```python
from build123d import *

# Parameters (mm, degrees)
SKETCH1_R               = 8.382
BOSS_EXTRUDE1_DEPTH     = 7.62
SKETCH2_R               = 5.588
BOSS_EXTRUDE2_DEPTH     = 7.112
SKETCH3_R               = 8.382
BOSS_EXTRUDE3_DEPTH     = 1.27
SKETCH4_R               = 2.54
CUT_EXTRUDE1_DEPTH      = 1
CUT_EXTRUDE1_DEPTH_BACK = 17.002
CHAMFER1_SIZE           = 0.508
SKETCH5_R               = 1.651
CUT_EXTRUDE2_DEPTH      = 9.382


with BuildPart() as part:
    # Sketch1 → Boss-Extrude1 (new body)
    with BuildSketch(Plane(origin=(0, 0, 0), x_dir=(1, 0, 0), z_dir=(0, 1, 0))):
        Circle(SKETCH1_R)
    extrude(amount=-BOSS_EXTRUDE1_DEPTH)

    # Sketch2 → Boss-Extrude2 (add)
    with BuildSketch(Plane(origin=(0, 0, 0), x_dir=(1, 0, 0), z_dir=(0, 1, 0))):
        with BuildLine():
            ThreePointArc((-4.121307864, 3.77366738), (-4.666752119, 3.721610627), (-4.596130935, 3.178258081))
            ThreePointArc((-4.596130935, 3.178258081), (-4.368874324, 3.484061013), (-4.121307864, 3.77366738))
        make_face()
        with BuildLine():
            ThreePointArc((-4.857698061, 2.761976385), (-5.377883173, 2.589852039), (-5.188125293, 2.075837167))
            ThreePointArc((-5.188125293, 2.075837167), (-5.034614034, 2.424542334), (-4.857698061, 2.761976385))
        make_face()
        with BuildLine():
            ThreePointArc((-5.350502993, 1.611788361), (-5.819344708, 1.328227455), (-5.519965385, 0.86932511))
            ThreePointArc((-5.519965385, 0.86932511), (-5.447897173, 1.243446979), (-5.350502993, 1.611788361))
        make_face()
        with BuildLine():
            ThreePointArc((-5.575011364, 0.380778538), (-5.969, 0), (-5.575011364, -0.380778538))
            ThreePointArc((-5.575011364, -0.380778538), (-5.588, 0), (-5.575011364, 0.380778538))
        make_face()
        with BuildLine():
            ThreePointArc((-5.350502993, -1.611788361), (-5.447897173, -1.243446979), (-5.519965385, -0.86932511))
            ThreePointArc((-5.519965385, -0.86932511), (-5.819344708, -1.328227455), (-5.350502993, -1.611788361))
        make_face()
        with BuildLine():
            ThreePointArc((-4.857698061, -2.761976385), (-5.034614034, -2.424542334), (-5.188125293, -2.075837167))
            ThreePointArc((-5.188125293, -2.075837167), (-5.377883173, -2.589852039), (-4.857698061, -2.761976385))
        make_face()
        with BuildLine():
            ThreePointArc((-4.121307864, -3.77366738), (-4.368874324, -3.484061013), (-4.596130935, -3.178258081))
            ThreePointArc((-4.596130935, -3.178258081), (-4.666752119, -3.721610627), (-4.121307864, -3.77366738))
        make_face()
        with BuildLine():
            ThreePointArc((-2.075837167, -5.188125293), (-2.424542334, -5.034614034), (-2.761976385, -4.857698061))
            ThreePointArc((-2.761976385, -4.857698061), (-2.589852039, -5.377883173), (-2.075837167, -5.188125293))
        make_face()
        with BuildLine():
            ThreePointArc((-0.86932511, -5.519965385), (-1.243446979, -5.447897173), (-1.611788361, -5.350502993))
            ThreePointArc((-1.611788361, -5.350502993), (-1.328227455, -5.819344708), (-0.86932511, -5.519965385))
        make_face()
        with BuildLine():
            ThreePointArc((2.761976385, -4.857698061), (2.424542334, -5.034614034), (2.075837167, -5.188125293))
            ThreePointArc((2.075837167, -5.188125293), (2.589852039, -5.377883173), (2.761976385, -4.857698061))
        make_face()
        with BuildLine():
            ThreePointArc((3.77366738, -4.121307864), (3.484061013, -4.368874324), (3.178258081, -4.596130935))
            ThreePointArc((3.178258081, -4.596130935), (3.721610627, -4.666752119), (3.77366738, -4.121307864))
        make_face()
        with BuildLine():
            ThreePointArc((4.596130935, -3.178258081), (4.368874324, -3.484061013), (4.121307864, -3.77366738))
            ThreePointArc((4.121307864, -3.77366738), (4.666752119, -3.721610627), (4.596130935, -3.178258081))
        make_face()
        with BuildLine():
            ThreePointArc((5.188125293, -2.075837167), (5.034614034, -2.424542334), (4.857698061, -2.761976385))
            ThreePointArc((4.857698061, -2.761976385), (5.377883173, -2.589852039), (5.188125293, -2.075837167))
        make_face()
        with BuildLine():
            ThreePointArc((5.588, 0), (5.584751897, -0.1905), (5.575011364, -0.380778538))
            ThreePointArc((5.575011364, -0.380778538), (5.969, 0), (5.575011364, 0.380778538))
            ThreePointArc((5.575011364, 0.380778538), (5.584751897, 0.1905), (5.588, 0))
        make_face()
        with BuildLine():
            ThreePointArc((5.519965385, 0.86932511), (5.819344708, 1.328227455), (5.350502993, 1.611788361))
            ThreePointArc((5.350502993, 1.611788361), (5.447897173, 1.243446979), (5.519965385, 0.86932511))
        make_face()
        with BuildLine():
            ThreePointArc((5.188125293, 2.075837167), (5.377883173, 2.589852039), (4.857698061, 2.761976385))
            ThreePointArc((4.857698061, 2.761976385), (5.034614034, 2.424542334), (5.188125293, 2.075837167))
        make_face()
        with BuildLine():
            ThreePointArc((4.596130935, 3.178258081), (4.666752119, 3.721610627), (4.121307864, 3.77366738))
            ThreePointArc((4.121307864, 3.77366738), (4.368874324, 3.484061013), (4.596130935, 3.178258081))
        make_face()
        with BuildLine():
            ThreePointArc((3.77366738, 4.121307864), (3.721610627, 4.666752119), (3.178258081, 4.596130935))
            ThreePointArc((3.178258081, 4.596130935), (3.484061013, 4.368874324), (3.77366738, 4.121307864))
        make_face()
        with BuildLine():
            ThreePointArc((2.761976385, 4.857698061), (2.589852039, 5.377883173), (2.075837167, 5.188125293))
            ThreePointArc((2.075837167, 5.188125293), (2.424542334, 5.034614034), (2.761976385, 4.857698061))
        make_face()
        with BuildLine():
            ThreePointArc((1.611788361, 5.350502993), (1.328227455, 5.819344708), (0.86932511, 5.519965385))
            ThreePointArc((0.86932511, 5.519965385), (1.243446979, 5.447897173), (1.611788361, 5.350502993))
        make_face()
        with BuildLine():
            ThreePointArc((0.380778538, 5.575011364), (0, 5.969), (-0.380778538, 5.575011364))
            ThreePointArc((-0.380778538, 5.575011364), (0, 5.588), (0.380778538, 5.575011364))
        make_face()
        with BuildLine():
            ThreePointArc((-0.86932511, 5.519965385), (-1.328227455, 5.819344708), (-1.611788361, 5.350502993))
            ThreePointArc((-1.611788361, 5.350502993), (-1.243446979, 5.447897173), (-0.86932511, 5.519965385))
        make_face()
        with BuildLine():
            ThreePointArc((-2.075837167, 5.188125293), (-2.589852039, 5.377883173), (-2.761976385, 4.857698061))
            ThreePointArc((-2.761976385, 4.857698061), (-2.424542334, 5.034614034), (-2.075837167, 5.188125293))
        make_face()
        with BuildLine():
            ThreePointArc((-3.178258081, 4.596130935), (-3.721610627, 4.666752119), (-3.77366738, 4.121307864))
            ThreePointArc((-3.77366738, 4.121307864), (-3.484061013, 4.368874324), (-3.178258081, 4.596130935))
        make_face()
        with BuildLine():
            ThreePointArc((-3.178258081, -4.596130935), (-3.484061013, -4.368874324), (-3.77366738, -4.121307864))
            ThreePointArc((-3.77366738, -4.121307864), (-3.721610627, -4.666752119), (-3.178258081, -4.596130935))
        make_face()
        with BuildLine():
            ThreePointArc((0.380778538, -5.575011364), (0, -5.588), (-0.380778538, -5.575011364))
            ThreePointArc((-0.380778538, -5.575011364), (0, -5.969), (0.380778538, -5.575011364))
        make_face()
        with BuildLine():
            ThreePointArc((1.611788361, -5.350502993), (1.243446979, -5.447897173), (0.86932511, -5.519965385))
            ThreePointArc((0.86932511, -5.519965385), (1.328227455, -5.819344708), (1.611788361, -5.350502993))
        make_face()
        with BuildLine():
            ThreePointArc((5.519965385, -0.86932511), (5.447897173, -1.243446979), (5.350502993, -1.611788361))
            ThreePointArc((5.350502993, -1.611788361), (5.819344708, -1.328227455), (5.519965385, -0.86932511))
        make_face()
        Circle(SKETCH2_R)
    extrude(amount=BOSS_EXTRUDE2_DEPTH)

    # Sketch3 → Boss-Extrude3 (add)
    with BuildSketch(Plane(origin=(0, 7.112, 0), x_dir=(1, 0, 0), z_dir=(0, 1, 0))):
        Circle(SKETCH3_R)
    extrude(amount=BOSS_EXTRUDE3_DEPTH)

    # Sketch4 → Cut-Extrude1 (cut, two sides)
    with BuildSketch(Plane.XZ.offset(7.62)) as cut_extrude1_sk:
        Circle(SKETCH4_R)
    extrude(amount=CUT_EXTRUDE1_DEPTH, mode=Mode.SUBTRACT)
    extrude(cut_extrude1_sk.sketch, amount=-CUT_EXTRUDE1_DEPTH_BACK, mode=Mode.SUBTRACT)

    # Chamfer1
    chamfer1_edges = [part.edges().sort_by_distance(p)[0] for p in [
        (-2.54, 8.382, 0),
        (-2.54, -7.62, 0),
    ]]
    chamfer(chamfer1_edges, length=CHAMFER1_SIZE)

    # Sketch5 → Cut-Extrude2 (cut, through all)
    with BuildSketch(Plane(origin=(0, 0, 0), x_dir=(0, 0, -1), z_dir=(1, 0, 0))):
        with Locations((0, -3.81)):
            Circle(SKETCH5_R)
    extrude(amount=-CUT_EXTRUDE2_DEPTH, mode=Mode.SUBTRACT)


solid = part.part
```
Verification items for the finished model (mm, model axes). A direction names the side the tool comes from. Round coordinates to 2 decimals unless told otherwise and drop trailing zeros. Order: outer loops, then holes, each group sorted by start corner. A loop starts at its lowest first (then second) coordinate and runs counter-clockwise, first axis right, second up.
1) Cross-section at A-A, the plane z = 0. Record the cut outline in (x, y), plus the area to 3 significant figures.
Geometry says:
outline: (-8.38, -7.62) - (-3.05, -7.62) - (-2.54, -7.11) - (-2.54, -5.46) - (-8.38, -5.46) - close; (-8.38, -2.16) - (-2.54, -2.16) - (-2.54, 7.87) - (-3.05, 8.38) - (-8.38, 8.38) - (-8.38, 7.11) - (-5.97, 7.11) - (-5.97, 0) - (-8.38, 0) - close; (2.54, -7.11) - (3.05, -7.62) - (8.38, -7.62) - (8.38, 0) - (5.97, 0) - (5.97, 7.11) - (8.38, 7.11) - (8.38, 8.38) - (3.05, 8.38) - (2.54, 7.87) - close
area: 133 mm2
2) Tool access check on faces 5 (the cylindrical face through (7.743, -3.757, 3.21)), 6 (the cylindrical face through (-5.11, -3.74, 1.65)). Record the directions out of +Z, -Z, +X, -X, +Y, -Y that give a thin tool (end or side, any length) a straight path to the whole face; none if there is none.
Geometry says:
face 5: +Y, -Y
face 6: -X
3) Depth check by flat-ended pin: pin 1 (3 mm diameter, centred on y = -3, z = 5, fed in from +X); pin 2 (1 mm diameter, centred on y = -6, z = -3, fed in from -X); pin 3 (5 mm diameter, centred on x = 3, y = -0.5, fed in from -Z). Enter the tip coordinate at first touch or a pass-through.
Geometry says:
pin 1: stops at x = 7.62
pin 2: stops at x = -8
pin 3: stops at z = -8.37
4) Cross-section at D-D, the plane x = 7. Record the cut outline in (y, z).
Geometry says:
outline: (-7.62, -4.61) - (0, -4.61) - (0, 4.61) - (-7.62, 4.61) - close; (7.11, -4.61) - (8.38, -4.61) - (8.38, 4.61) - (7.11, 4.61) - close
5) Draft check along Y on faces 1 (the flat face through (-2, 7.112, 5.5)), 2 (the flat face through (-2, 0, 5.5)), 3 (the flat face through (0, -7.62, 4)), 4 (the flat face through (0, 8.382, 4)). Enter one of: +Y half, -Y half, draft (parallel to the pull), parting line (faces both ways), or undercut.
Geometry says:
face 1: undercut
face 2: undercut
face 3: -Y half
face 4: +Y half
6) Material ranges on line 1 (Z direction, x = 0, y = -2.75); line 2 (Z direction, x = 0, y = 0.75), recorded low to high.
Geometry says:
line 1: z = -8.38 to -2.54, 2.54 to 8.38
line 2: z = -5.97 to -2.54, 2.54 to 5.97
7) Cross-section at C-C, the plane y = -3.81. Record the cut outline in (x, z).
Geometry says:
outline: (-8.22, -1.65) arc R8.38 ccw (long way) to (-8.22, 1.65) - (-1.93, 1.65) arc R2.54 cw (long way) to (-1.93, -1.65) - close
8) Cross-section at B-B, the plane x = 0. Record the cut outline in (y, z), plus the area to 3 significant figures.
Geometry says:
outline: (-7.62, -8.38) - (0, -8.38) - (0, -5.97) - (7.11, -5.97) - (7.11, -8.38) - (8.38, -8.38) - (8.38, -3.05) - (7.87, -2.54) - (-7.11, -2.54) - (-7.62, -3.05) - close; (-7.62, 3.05) - (-7.11, 2.54) - (7.87, 2.54) - (8.38, 3.05) - (8.38, 8.38) - (7.11, 8.38) - (7.11, 5.97) - (0, 5.97) - (0, 8.38) - (-7.62, 8.38) - close
area: 152 mm2
